```python
from build123d import *

# Parameters (mm, degrees)
SKETCH1_W           = 6.35
SKETCH1_H           = 9
SKETCH1_R           = 1.591
BOSS_EXTRUDE1_DEPTH = 30
SKETCH2_R           = 1.59
CUT_EXTRUDE1_DEPTH  = 30


with BuildPart() as part:
    # Sketch1 → Boss-Extrude1 (new body)
    with BuildSketch(Plane.XY):
        with Locations((3.175, -4.5)):
            Rectangle(SKETCH1_W, SKETCH1_H)
        with Locations((3.175, -6.5)):
            Circle(SKETCH1_R, mode=Mode.SUBTRACT)
    extrude(amount=BOSS_EXTRUDE1_DEPTH)

    # Sketch2 → Cut-Extrude1 (cut)
    with BuildSketch(Plane(origin=(0, 0, 0), x_dir=(0, 0, -1), z_dir=(1, 0, 0))):
        with Locations(Location((-24, -3, 0), (0, 0, 270))):
            Circle(SKETCH2_R)
        with Locations(Location((-6, -3, 0), (0, 0, 270))):
            Circle(SKETCH2_R)
    extrude(amount=CUT_EXTRUDE1_DEPTH, mode=Mode.SUBTRACT)


solid = part.part
```
Geometry check sheet. Reference: the model listing, model coordinates, mm. Give positions to 0.01 mm unless a question says otherwise; leave off trailing zeros. Order: outer loops, then holes, each group sorted by start corner. A loop starts at its lowest first (then second) coordinate and runs counter-clockwise, first axis right, second up. Notation, with made-up numbers: (41.25, 22) - (72.25, 22) arc R24 ccw to (72.25, 41) - close; hole circle Ø9 at (20.25, 49). An arc over 180 degrees is marked (long way). Write item = value, one per line. Start each with the question number.
1) Section check D-D (y = -6.5). Enter the section's corners in (x, z).
2) Section check C-C (x = 4.5). Enter the section's corners in (y, z), then the cut area to 3 significant figures.
3) Section check A-A (z = 6). Enter the section's corners in (x, y) (3 decimals).
4) Scan lines: L1, parallel to Z at x = 4, y = -3; L2, parallel to Z at x = 1.75, y = -4.25; L3, parallel to Y at x = 3.5, z = 6. Record each from-to range of solid material in increasing order.
5) Draft check along Y on faces 1 (the cylindrical face through (3.131, -2.793, 4.424)), 2 (the flat face through (3, -4, 30)), 3 (the flat face through (3, 0, 15)), 4 (the flat face through (3, -9, 15)). Enter one of: released by +Y, released by -Y, zero draft, split by the parting line, or undercut.
6) Section check B-B (y = -3.25). Enter the section's corners in (x, z), then the cut area to 3 significant figures.
Geometry check:
q1.outline = (0, 0) - (1.58, 0) - (1.58, 30) - (0, 30) - close; (4.77, 0) - (6.35, 0) - (6.35, 30) - (4.77, 30) - close
q2.outline = (-9, 0) - (-7.38, 0) - (-7.38, 30) - (-9, 30) - close; (-5.62, 0) - (0, 0) - (0, 30) - (-5.62, 30) - close; hole circle Ø3.18 at (-3, 6); hole circle Ø3.18 at (-3, 24)
q2.area = 201 mm2
q3.outline = (0, -9) - (6.35, -9) - (6.35, -4.59) - (0, -4.59) - close; (0, -1.41) - (6.35, -1.41) - (6.35, 0) - (0, 0) - close; hole circle Ø3.182 at (3.175, -6.5)
q4.L1 = 0 to 4.41, 7.59 to 22.41, 25.59 to 30
q4.L2 = 0 to 5.02, 6.98 to 23.02, 24.98 to 30
q4.L3 = -9 to -8.06, -4.94 to -4.59, -1.41 to 0
q5.face_1 = undercut
q5.face_2 = zero draft
q5.face_3 = released by +Y
q5.face_4 = released by -Y
q6.outline = (0, 0) - (6.35, 0) - (6.35, 4.43) - (0, 4.43) - close; (0, 7.57) - (6.35, 7.57) - (6.35, 22.43) - (0, 22.43) - close; (0, 25.57) - (6.35, 25.57) - (6.35, 30) - (0, 30) - close
q6.area = 151 mm2
